Autodesk Inventor part; units mm, degrees
ref_plane "YZ Plane" through (0, 0, 0) normal (1, 0, 0) x (0, 1, 0)
ref_plane "XZ Plane" through (0, 0, 0) normal (0, 1, 0) x (-1, 0, 0)
ref_plane "XY Plane" through (0, 0, 0) normal (0, 0, 1) x (1, 0, 0)
sketch "Sketch3" plane through (0, 0, 0) normal (0, 1, 0) x (-1, 0, 0)
  line L0 (0, 0) -> (9, 0)
  line L1 (9, 0) -> (9, -3)
  line L2 (9, -3) -> (0, -3)
  line L3 (0, -3) -> (0, 0)
  line L4 (0, 1) -> (12, 1)
  line L5 (12, 1) -> (12, -9)
  line L6 (12, -9) -> (-3, -9)
  line L7 (0, 1) -> (-3, 1)
  line L8 (-3, 1) -> (-3, -9)
  dimension "d17" = 3
  dimension "d19" = 12
  dimension "d20" = 10
extrude "Extrusion3" add sketch "Sketch3" along normal blind 10
sketch "Sketch4" plane through (0, 10, 0) normal (0, 1, 0) x (1, 0, 0)
  line L0 (-12, 9) -> (-12, -1)
  line L1 (3, 9) -> (-12, 9)
  line L2 (3, -1) -> (3, 9)
  line L3 (-12, -1) -> (3, -1)
  point P0 (0, 0)
extrude "Extrusion4" add sketch "Sketch4" along normal blind 2
properties part number "reed-switch-design-test"
The listing builds one solid part. Answer for the finished solid, in the listing's coordinates (mm). A direction names the side the tool comes from. Coordinates: 2 decimals unless noted, no trailing zeros. Write each loop counter-clockwise with the first axis right and the second up, starting at its lowest first coordinate (ties: lowest second). Pieces come first, ordered by that corner, then holes. Notation, with made-up numbers: (-32, 61.25) - (22, 61.25) arc R15 cw to (22, 87.25) - close; hole circle Ø7 at (36.5, -12). An arc over 180 degrees is marked (long way). Return JSON: item names as keys, results as strings. Group by question number.
Q1. Which of the six approach directions +Z, -Z, +X, -X, +Y, -Y give full straight-line access (tool end or side, diameter ignored) to faces 1 (the flat face through (-4, 5, 0)), 2 (the flat face through (3, 6, -4))?
Q2. The part is cut by section B-B on x = -6.25. Write down the section's boundary in (y, z), and give its area (3 significant figures).
Q3. The part is cut by section C-C on z = -2.5. Write down the section's boundary in (x, y), and give its area (3 significant figures).
Q4. For a pull along X with two mould halves and no side action, classify faces 3 (the flat face through (-4, 0, -4)), 4 (the flat face through (-5, 10, -2)), 5 (the flat face through (-12, 6, -4)) as +X half, -X half, draft (parallel to the pull), parting line (faces both ways), or undercut.
Q5. Find the intervals of material crossed by line 1 along Z through (x, y) = (-6.5, 5.25); line 2 along X through (y, z) = (5.75, -0.75); line 3 along Y through (x, z) = (-8.5, -1.75), in increasing order. Write a range as [from, to].
Q6. The part is cut by section A-A on y = 9.5. Write down the section's boundary in (x, z), and give its area (3 significant figures).
Evaluation:
{
 "1": {"face 1": "-Y", "face 2": "+Z, -Z, +X, +Y, -Y"},
 "2": {"outline": "(0, -9) - (12, -9) - (12, 1) - (0, 1) - (0, 0) - (10, 0) - (10, -3) - (0, -3) - close", "area": "90.0 mm2"},
 "3": {"outline": "(-12, 0) - (-9, 0) - (-9, 10) - (0, 10) - (0, 0) - (3, 0) - (3, 12) - (-12, 12) - close", "area": "90.0 mm2"},
 "4": {"face 3": "draft", "face 4": "undercut", "face 5": "-X half"},
 "5": {"line 1": "z = [-9, -3], [0, 1]", "line 2": "x = [-12, -9], [0, 3]", "line 3": "y = [10, 12]"},
 "6": {"outline": "(-12, -9) - (3, -9) - (3, 1) - (-12, 1) - close; hole (-9, -3) - (0, -3) - (0, 0) - (-9, 0) - close", "area": "123 mm2"}
}
